from build123d import *
from OCP.BRepFilletAPI import BRepFilletAPI_MakeChamfer

# Parameters (mm, degrees)
DODANIE_WYCI_GNI_CIE2_DEPTH = 4
WYTNIJ_WYCI_GNI_CIE3_START  = -1
WYTNIJ_WYCI_GNI_CIE3_DEPTH  = 34.205262753
SZKIC6_3_R                  = 3.6
WYTNIJ_WYCI_GNI_CIE4_DEPTH  = 35.205262753
DODANIE_WYCI_GNI_CIE3_DEPTH = 24.5
DODANIE_WYCI_GNI_CIE4_DEPTH = 46
DODANIE_WYCI_GNI_CIE5_DEPTH = 70.5
SFAZOWANIE3_SIZE            = 0.7
ZAOKR_GLENIE1_R             = 1
ZAOKR_GLENIE2_R             = 5
WYTNIJ_WYCI_GNI_CIE1_REACH  = 86.592
SZKIC3_W                    = 18
SZKIC3_H                    = 3.5
SFAZOWANIE1_SIZE            = 2.5
SFAZOWANIE1_SIZE2           = 4.330127019
ZAOKR_GLENIE4_R             = 2
SFAZOWANIE2_SIZE            = 1
ZAOKR_GLENIE3_R             = 5
SZKIC10_R                   = 2.1
WYTNIJ_WYCI_GNI_CIE5_DEPTH  = 82.189531345
SZYK_KO_OWY1_COUNT          = 4
SZKIC12_R                   = 1.65
WYTNIJ_WYCI_GNI_CIE6_DEPTH  = 91.228653985


# Read off the part's stored shape, not the designer's step: Lustro1
# Some blends are built 0.0001 mm under size
with BuildPart() as part:
    # Szkic1 → Dodanie-wyciągnięcie2 (new body)
    with BuildSketch(Plane(origin=(0, 0, 0), x_dir=(1, 0, 0), z_dir=(0, 1, 0))):
        Polygon((-25, -21), (-25, -22), (25, -22), (25, -21), (25, 23), (-25, 23), align=None)
    extrude(amount=DODANIE_WYCI_GNI_CIE2_DEPTH)

    # Szkic6 → Wytnij-wyciągnięcie3 (cut, through all)
    with BuildSketch(Plane(origin=(0, 4, 0), x_dir=(1, 0, 0), z_dir=(0, 1, 0)).offset(WYTNIJ_WYCI_GNI_CIE3_START)):
        with BuildLine():
            Line((-12.02081528, -7.778174593), (-17.67766953, -13.435028843))
            ThreePointArc((-17.67766953, -13.435028843), (-17.67766953, -17.67766953), (-13.435028843, -17.67766953))
            Line((-13.435028843, -17.67766953), (-7.778174593, -12.02081528))
            ThreePointArc((-7.778174593, -12.02081528), (-7.778174593, -7.778174593), (-12.02081528, -7.778174593))
        make_face()
        with BuildLine():
            Line((-7.778174593, 12.02081528), (-13.435028843, 17.67766953))
            ThreePointArc((-13.435028843, 17.67766953), (-17.67766953, 17.67766953), (-17.67766953, 13.435028843))
            Line((-17.67766953, 13.435028843), (-12.02081528, 7.778174593))
            ThreePointArc((-12.02081528, 7.778174593), (-7.778174593, 7.778174593), (-7.778174593, 12.02081528))
        make_face()
        with BuildLine():
            Line((12.02081528, 7.778174593), (17.67766953, 13.435028843))
            ThreePointArc((17.67766953, 13.435028843), (17.67766953, 17.67766953), (13.435028843, 17.67766953))
            Line((13.435028843, 17.67766953), (7.778174593, 12.02081528))
            ThreePointArc((7.778174593, 12.02081528), (7.778174593, 7.778174593), (12.02081528, 7.778174593))
        make_face()
        with BuildLine():
            Line((7.778174593, -12.02081528), (13.435028843, -17.67766953))
            ThreePointArc((13.435028843, -17.67766953), (17.67766953, -17.67766953), (17.67766953, -13.435028843))
            Line((17.67766953, -13.435028843), (12.02081528, -7.778174593))
            ThreePointArc((12.02081528, -7.778174593), (7.778174593, -7.778174593), (7.778174593, -12.02081528))
        make_face()
    extrude(amount=-WYTNIJ_WYCI_GNI_CIE3_DEPTH, mode=Mode.SUBTRACT)

    # Szkic6<3> → Wytnij-wyciągnięcie4 (cut, through all)
    with BuildSketch(Plane(origin=(0, 4, 0), x_dir=(1, 0, 0), z_dir=(0, 1, 0))):
        with Locations(Location((0, 0, 0), (0, 0, 270))):
            Circle(SZKIC6_3_R)
    extrude(amount=-WYTNIJ_WYCI_GNI_CIE4_DEPTH, mode=Mode.SUBTRACT)

    # Szkic2 → Dodanie-wyciągnięcie3 (add)
    with BuildSketch(Plane.XZ):
        Polygon((15.7, -6.5), (15.7, 6.5), (25, 15.172390301), (25, -15.172390301), align=None)
    extrude(amount=DODANIE_WYCI_GNI_CIE3_DEPTH)

    # Szkic8 → Dodanie-wyciągnięcie4 (add)
    with BuildSketch(Plane.XZ.offset(24.5)):
        Polygon((25, 15.172390301), (25, -15.172390301), (22.7, -13.027605603), (22.7, 13.027605603), align=None)
    extrude(amount=DODANIE_WYCI_GNI_CIE4_DEPTH)

    # Szkic11 → Dodanie-wyciągnięcie5 (add)
    with BuildSketch(Plane.XZ.offset(70.5)):
        Polygon((25, 15.172390301), (25, -15.172390301), (25.7, -13.711437924), (25.7, 13.711439266), align=None)
    extrude(amount=-DODANIE_WYCI_GNI_CIE5_DEPTH)

    # Sfazowanie3
    sfazowanie3_edges = [part.edges().sort_by_distance(p)[0] for p in [
        (25.7, 0, 6.71e-07),
    ]]
    chamfer(sfazowanie3_edges, length=SFAZOWANIE3_SIZE - 0.0001)  # a hair under: the kernel refuses the full size

    # Zaokrąglenie1
    # the kernel refuses this fillet: 1 mm, written as the material it takes off along each edge
    with BuildSketch(Plane(origin=(25, 0, 15.172390301), x_dir=(0.4321005826211705, 0, -0.9018254190797934), z_dir=(0, -1, 0))) as zaokr_glenie1_piece_1:
        with BuildLine():
            CenterArc((ZAOKR_GLENIE1_R * 1.36131157072, -ZAOKR_GLENIE1_R), ZAOKR_GLENIE1_R, 90, 107.399057565)
            Line((ZAOKR_GLENIE1_R * 0.407066323534, -ZAOKR_GLENIE1_R * 1.2990250963), (0, 0))
            Line((0, 0), (ZAOKR_GLENIE1_R * 1.36131157072, 0))
        make_face()
    extrude(amount=73.903278927, mode=Mode.SUBTRACT)
    with BuildSketch(Plane(origin=(25, -73.903280204, -15.172390301), x_dir=(0.43210025968346966, 0, 0.901825573812075), z_dir=(0, 1, 0))) as zaokr_glenie1_piece_2:
        with BuildLine():
            CenterArc((ZAOKR_GLENIE1_R * 1.36131208157, -ZAOKR_GLENIE1_R), ZAOKR_GLENIE1_R, 90, 107.399078082)
            Line((ZAOKR_GLENIE1_R * 0.407066941463, -ZAOKR_GLENIE1_R * 1.29902543801), (0, 0))
            Line((0, 0), (ZAOKR_GLENIE1_R * 1.36131208157, 0))
        make_face()
    extrude(amount=73.903280204, mode=Mode.SUBTRACT)

    # Zaokrąglenie2
    zaokr_glenie2_edges = [part.edges().sort_by_distance(p)[0] for p in [
        (15.7, -12.25, 6.5),
        (15.7, -12.25, -6.5),
    ]]
    fillet(zaokr_glenie2_edges, radius=ZAOKR_GLENIE2_R)

    # Szkic3 → Wytnij-wyciągnięcie1 (cut, up to next)
    with BuildSketch(Plane.ZY.offset(-15.7), mode=Mode.PRIVATE) as wytnij_wyci_gni_cie1_sk1:
        with Locations((0, -11.75)):
            Rectangle(SZKIC3_W, SZKIC3_H)
    wytnij_wyci_gni_cie1_tool1 = extrude(wytnij_wyci_gni_cie1_sk1.sketch, amount=-WYTNIJ_WYCI_GNI_CIE1_REACH, mode=Mode.PRIVATE) & part.part
    add(wytnij_wyci_gni_cie1_tool1.solids().sort_by_distance((15.7, -11.75, 0))[0], mode=Mode.SUBTRACT)

    # Sfazowanie1: one chamfer whose edges measure the first distance from different faces: ONE call of the kernel's chamfer builder (chamfer() names one face for all edges)
    sfazowanie1_edges_1 = [part.edges().sort_by_distance(p)[0] for p in [
        (22.040460888, -13.5, -9),
    ]]
    sfazowanie1_side_1 = [part.faces().sort_by_distance(p)[0] for p in [
        (22.040460888, -11.75, -9),
    ]]
    sfazowanie1_edges_2 = [part.edges().sort_by_distance(p)[0] for p in [
        (22.040460888, -13.5, 9),
    ]]
    sfazowanie1_side_2 = [part.faces().sort_by_distance(p)[0] for p in [
        (22.040460888, -11.75, 9),
    ]]
    sfazowanie1 = BRepFilletAPI_MakeChamfer(part.part.solid().wrapped)
    for e in sfazowanie1_edges_1:
        sfazowanie1.Add(SFAZOWANIE1_SIZE, SFAZOWANIE1_SIZE2, e.wrapped, sfazowanie1_side_1[0].wrapped)  # the first distance lies on this face
    for e in sfazowanie1_edges_2:
        sfazowanie1.Add(SFAZOWANIE1_SIZE, SFAZOWANIE1_SIZE2, e.wrapped, sfazowanie1_side_2[0].wrapped)  # the first distance lies on this face
    add(Compound.cast(sfazowanie1.Shape()), mode=Mode.REPLACE)

    # Zaokrąglenie4
    zaokr_glenie4_edges = [part.edges().sort_by_distance(p)[0] for p in [
        (22.7, -24.5, 0),
    ]]
    fillet(zaokr_glenie4_edges, radius=ZAOKR_GLENIE4_R)

    # Lustro1: part across plane


with BuildPart() as part_1:
    add(part.part)
    add(part.part.mirror(Plane(origin=(0, 0, 0), x_dir=(0, 0, 1), z_dir=(1, 0, 0))))

    # Sfazowanie2
    sfazowanie2_edges = [part_1.edges().sort_by_distance(p)[0] for p in [
        (25.7, -13.5, 0),
        (25.7, -12.25, -6.834936491),
        (25.7, -12.25, 6.834936491),
        (-25.7, -13.5, 0),
        (-25.7, -12.25, -6.834936491),
        (-25.7, -12.25, 6.834936491),
    ]]
    chamfer(sfazowanie2_edges, length=SFAZOWANIE2_SIZE)

    # Zaokrąglenie3
    zaokr_glenie3_edges = [part_1.edges().sort_by_distance(p)[0] for p in [
        (25, 2, 22),
        (-25, 2, 22),
        (-25, 2, -23),
        (25, 2, -23),
    ]]
    fillet(zaokr_glenie3_edges, radius=ZAOKR_GLENIE3_R)

    # Szkic10 → Wytnij-wyciągnięcie5 (cut, through all)
    with BuildSketch(Plane.XZ.offset(-3)):
        with Locations(Location((-15.556349186, 15.556349186, 0), (0, 0, 270))):
            Circle(SZKIC10_R)
    wytnij_wyci_gni_cie5 = extrude(amount=-WYTNIJ_WYCI_GNI_CIE5_DEPTH, mode=Mode.SUBTRACT)

    # Szyk kołowy1: Wytnij-wyciągnięcie5 ×4 about axis
    szyk_ko_owy1_axis = Axis((0, 0, 0), (0, 1, 0))
    for i in range(1, SZYK_KO_OWY1_COUNT):
        add(wytnij_wyci_gni_cie5.rotate(szyk_ko_owy1_axis, i * 360 / SZYK_KO_OWY1_COUNT), mode=Mode.SUBTRACT)

    # Szkic12 → Wytnij-wyciągnięcie6 (cut, through all)
    with BuildSketch(Plane.ZY.offset(25.7)):
        with Locations((8.711439266, -67)):
            Circle(SZKIC12_R)
        with Locations(Location((-8.711439266, -67, 0), (0, 0, 180))):
            Circle(SZKIC12_R)
    extrude(amount=-WYTNIJ_WYCI_GNI_CIE6_DEPTH, mode=Mode.SUBTRACT)


solid = part_1.part
CAD build for the part. Positions are in the model's coordinates, mm. A direction names the side the tool comes from. Coordinates: 2 decimals unless noted, no trailing zeros. Loops run counter-clockwise (first coordinate to the right, second up) from the corner with the lowest first, then second, coordinate; pieces in that order, holes last. Notation, with made-up numbers: (48.5, -27) -> (86.5, -27) arc R11 cw to (86.5, -16) -> close; hole circle Ø7 at (-5.5, -29.75). An arc over 180 degrees is marked (long way). One line per item, written item: value.
1. Flat gauge pins, fed straight in: P1, Ø13, axis at x = -15.5, z = -13.5, coming from the -Y side; P2, Ø8, axis at x = -10.5, z = 10.5, coming from the -Y side; P3, Ø1.1, axis at x = 21.5, y = -11, coming from the -Z side. Where does each tip first touch, or does it go through?
Answers:
P1: stops at y = -24.89
P2: stops at y = 0
P3: stops at z = -12.42
2. Which spindle directions (+Z, -Z, +X, -X, +Y, -Y) get a long thin tool onto all of the face, cutting with end or side? Do faces 1 (the face through (-24.885, -34.756, 14.493)), 2 (the face through (-25.207, -12.738, -7.004)), 3 (the face through (14.89, 1.52, 10.65)), 4 (the face through (-18, -24.5, 0)). Say none if no direction does.
Answers:
face 1: +Z, -Y
face 2: -X
face 3: -Y
face 4: +Z, -Z, -Y
3. Pull direction X, two halves, no side cores. Call faces 5 (the face through (16.1, -18.13, 6.29)), 6 (the face through (24, 2, 20)), 7 (the face through (24.179, -68.464, 9.473)): pulls with the +X half, pulls with the -X half, needs draft (parallel to the pull), parting line crosses it, or undercut.
Answers:
face 5: undercut
face 6: pulls with the +X half
face 7: needs draft
4. Drill centre lines: line 1 (Z direction, x = 25, y = -67); line 2 (Z direction, x = 23.45, y = -67); line 3 (X direction, y = -48.5, z = 10). Where is each one in solid material? Low to high. Write a range as [from, to].
Answers:
line 1: z = [-14.46, -10.36], [-7.06, 7.06], [10.36, 14.46]
line 2: z = [-13.73, -10.36], [-7.06, 7.06], [10.36, 13.73]
line 3: x = [-25.7, -22.7], [22.7, 25.7]
5. Slice it at D-D on x = 2. Write the cut outline in (y, z), and give its area (3 significant figures).
Answers:
outline: (0, -23) -> (4, -23) -> (4, -2.99) -> (0, -2.99) -> close; (0, 2.99) -> (4, 2.99) -> (4, 22) -> (0, 22) -> close
area: 156 mm^2
6. Slice it at A-A on y = -67. Give the number of separate pieces and of enclosed holes in the cut face, and give its area (3 significant figures).
Answers:
separate pieces: 6
enclosed holes: 0
area: 129 mm^2
7. Slice it at C-C on y = -9. Write the cut outline in (x, z), and give its area (3 significant figures).
Answers:
outline: (-25.7, -13.71) -> (-25.59, -13.94) arc R1 ccw to (-24, -14.24) -> (-17.29, -7.98) arc R5 ccw to (-15.7, -4.33) -> (-15.7, 4.33) arc R5 ccw to (-17.29, 7.98) -> (-24, 14.24) arc R1 ccw to (-25.59, 13.94) -> (-25.7, 13.71) -> close; (15.7, -4.33) arc R5 ccw to (17.29, -7.98) -> (24, -14.24) arc R1 ccw to (25.59, -13.94) -> (25.7, -13.71) -> (25.7, 13.71) -> (25.59, 13.94) arc R1 ccw to (24, 14.24) -> (17.29, 7.98) arc R5 ccw to (15.7, 4.33) -> close
area: 439 mm^2
